For this review, take the finished solid that the model builds, in its own axes (mm). Face numbers are marked on the shaded views. Coordinates: 2 decimals unless noted, no trailing zeros. Write each loop counter-clockwise with the first axis right and the second up, starting at its lowest first coordinate (ties: lowest second). Pieces come first, ordered by that corner, then holes. Notation, with made-up numbers: (59.5, 76.25) - (109.5, 76.25) arc R17 cw to (109.5, 82.25) - close; hole circle Ø4 at (63, 35.5). An arc over 180 degrees is marked (long way). Write each question's results on one line, items separated by ' | '.
from build123d import *

# Parameters (mm, degrees)
SKETCH1_R           = 2.25
BOSS_EXTRUDE1_DEPTH = 6
CUT_EXTRUDE1_DEPTH  = 11
FILLET1_R           = 2


with BuildPart() as part:
    # Sketch1 → Boss-Extrude1 (new body)
    with BuildSketch(Plane.XY):
        with BuildLine():
            Line((-5, 12), (-5, -5))
            Line((-5, -5), (5, -5))
            Line((5, -5), (5, 12))
            ThreePointArc((5, 12), (0, 17), (-5, 12))
        make_face()
        Circle(SKETCH1_R, mode=Mode.SUBTRACT)
    extrude(amount=BOSS_EXTRUDE1_DEPTH)

    # Sketch2 → Cut-Extrude1 (cut, through all)
    with BuildSketch(Plane(origin=(5, 0, 0), x_dir=(0, 0, -1), z_dir=(1, 0, 0))):
        Polygon((-6, 5), (-3, 17), (-6, 17), align=None)
    extrude(amount=-CUT_EXTRUDE1_DEPTH, mode=Mode.SUBTRACT)

    # Fillet1
    fillet1_edges = [part.edges().sort_by_distance(p)[0] for p in [
        (5, -5, 3),
        (-5, -5, 3),
    ]]
    fillet(fillet1_edges, radius=FILLET1_R)


solid = part.part
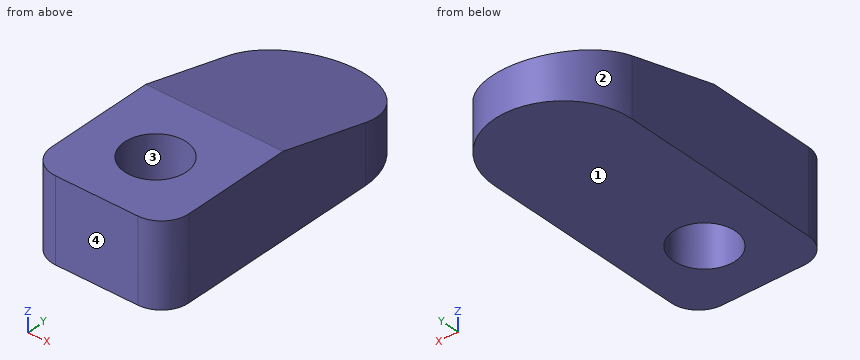
Q1. Wall thickness on line 1 along Y through (x, z) = (0, 1.65); line 2 along Z through (x, y) = (-3.25, 10.5) (3 decimals); line 3 along Y through (x, z) = (-3, 1.6): over which ranges is each line inside the solid? List them lowest first. Write a range as from..to.
Results found:
line 1: -5..-2.25, 2.25..17 | line 2: 0..4.625 | line 3: -5..16
Q2. Take a section at C-C on z = 4.45. State the section outline as (x, y) points.
Results found:
outline: (-5, -3) arc R2 ccw to (-3, -5) - (3, -5) arc R2 ccw to (5, -3) - (5, 11.2) - (-5, 11.2) - close; hole circle Ø4.5 at (0, 0)
Q3. Take a section at A-A on x = 0. State the section outline as (y, z) points.
Results found:
outline: (-5, 0) - (-2.25, 0) - (-2.25, 6) - (-5, 6) - close; (2.25, 0) - (17, 0) - (17, 3) - (5, 6) - (2.25, 6) - close
Q4. For pin 1 (6 mm diameter, centred on x = 1, y = 13, fed in from +Z), flat-tipped, find the tip position at first contact; note if it passes through.
Results found:
pin 1: z = 4.75
Q5. Take a section at D-D on z = 2.65. State the section outline as (x, y) points.
Results found:
outline: (-5, -3) arc R2 ccw to (-3, -5) - (3, -5) arc R2 ccw to (5, -3) - (5, 12) arc R5 ccw to (-5, 12) - close; hole circle Ø4.5 at (0, 0)
Q6. Take a section at B-B on y = 0. State the section outline as (x, z) points.
Results found:
outline: (-5, 0) - (-2.25, 0) - (-2.25, 6) - (-5, 6) - close; (2.25, 0) - (5, 0) - (5, 6) - (2.25, 6) - close
Q7. Mouldability with a two-part tool opening along Y and no side actions: class the marked faces 1, 2, 3 and 4 as pulls with the +Y half, pulls with the -Y half, needs draft (parallel to the pull), parting line crosses it, or undercut.
Results found:
face 1: needs draft | face 2: pulls with the +Y half | face 3: undercut | face 4: pulls with the -Y half
